from build123d import *

# Parameters (mm, degrees)
SKETCH3_R           = 3.9
BOSS_EXTRUDE1_DEPTH = 5
SKETCH5_R           = 3.6
BOSS_EXTRUDE2_DEPTH = 5
BOSS_EXTRUDE3_DEPTH = 5
SKETCH7_R           = 1.25
CUT_EXTRUDE1_DEPTH  = 11


with BuildPart() as part:
    # Sketch3 → Boss-Extrude1 (new body)
    with BuildSketch(Plane.XY):
        with Locations((10, 0)):
            Circle(SKETCH3_R)
        with BuildLine():
            Line((10, 2.1), (9.774921544, 2.489847322))
            ThreePointArc((9.774921544, 2.489847322), (9.608913837, 2.469220851), (9.444657197, 2.437538589))
            Line((9.444657197, 2.437538589), (9.351064312, 1.997218684))
            Line((9.351064312, 1.997218684), (9.016532531, 2.298432452))
            ThreePointArc((9.016532531, 2.298432452), (8.865023751, 2.22751631), (8.71859676, 2.146626594))
            Line((8.71859676, 2.146626594), (8.76565097, 1.698935688))
            Line((8.76565097, 1.698935688), (8.354412167, 1.882031))
            ThreePointArc((8.354412167, 1.882031), (8.232233047, 1.767766953), (8.117969, 1.645587833))
            Line((8.117969, 1.645587833), (8.301064312, 1.23434903))
            Line((8.301064312, 1.23434903), (7.853373406, 1.28140324))
            ThreePointArc((7.853373406, 1.28140324), (7.77248369, 1.134976249), (7.701567548, 0.983467469))
            Line((7.701567548, 0.983467469), (8.002781316, 0.648935688))
            Line((8.002781316, 0.648935688), (7.562461411, 0.555342803))
            ThreePointArc((7.562461411, 0.555342803), (7.530779149, 0.391086163), (7.510152678, 0.225078456))
            Line((7.510152678, 0.225078456), (7.9, 0))
            Line((7.9, 0), (7.510152678, -0.225078456))
            ThreePointArc((7.510152678, -0.225078456), (7.530779149, -0.391086163), (7.562461411, -0.555342803))
            Line((7.562461411, -0.555342803), (8.002781316, -0.648935688))
            Line((8.002781316, -0.648935688), (7.701567548, -0.983467469))
            ThreePointArc((7.701567548, -0.983467469), (7.77248369, -1.134976249), (7.853373406, -1.28140324))
            Line((7.853373406, -1.28140324), (8.301064312, -1.23434903))
            Line((8.301064312, -1.23434903), (8.117969, -1.645587833))
            ThreePointArc((8.117969, -1.645587833), (8.232233047, -1.767766953), (8.354412167, -1.882031))
            Line((8.354412167, -1.882031), (8.76565097, -1.698935688))
            Line((8.76565097, -1.698935688), (8.71859676, -2.146626594))
            ThreePointArc((8.71859676, -2.146626594), (8.865023751, -2.22751631), (9.016532531, -2.298432452))
            Line((9.016532531, -2.298432452), (9.351064312, -1.997218684))
            Line((9.351064312, -1.997218684), (9.444657197, -2.437538589))
            ThreePointArc((9.444657197, -2.437538589), (9.608913837, -2.469220851), (9.774921544, -2.489847322))
            Line((9.774921544, -2.489847322), (10, -2.1))
            Line((10, -2.1), (10.225078456, -2.489847322))
            ThreePointArc((10.225078456, -2.489847322), (10.391086163, -2.469220851), (10.555342803, -2.437538589))
            Line((10.555342803, -2.437538589), (10.648935688, -1.997218684))
            Line((10.648935688, -1.997218684), (10.983467469, -2.298432452))
            ThreePointArc((10.983467469, -2.298432452), (11.134976249, -2.22751631), (11.28140324, -2.146626594))
            Line((11.28140324, -2.146626594), (11.23434903, -1.698935688))
            Line((11.23434903, -1.698935688), (11.645587833, -1.882031))
            ThreePointArc((11.645587833, -1.882031), (11.767766953, -1.767766953), (11.882031, -1.645587833))
            Line((11.882031, -1.645587833), (11.698935688, -1.23434903))
            Line((11.698935688, -1.23434903), (12.146626594, -1.28140324))
            ThreePointArc((12.146626594, -1.28140324), (12.22751631, -1.134976249), (12.298432452, -0.983467469))
            Line((12.298432452, -0.983467469), (11.997218684, -0.648935688))
            Line((11.997218684, -0.648935688), (12.437538589, -0.555342803))
            ThreePointArc((12.437538589, -0.555342803), (12.469220851, -0.391086163), (12.489847322, -0.225078456))
            Line((12.489847322, -0.225078456), (12.1, 0))
            Line((12.1, 0), (12.489847322, 0.225078456))
            ThreePointArc((12.489847322, 0.225078456), (12.469220851, 0.391086163), (12.437538589, 0.555342803))
            Line((12.437538589, 0.555342803), (11.997218684, 0.648935688))
            Line((11.997218684, 0.648935688), (12.298432452, 0.983467469))
            ThreePointArc((12.298432452, 0.983467469), (12.22751631, 1.134976249), (12.146626594, 1.28140324))
            Line((12.146626594, 1.28140324), (11.698935688, 1.23434903))
            Line((11.698935688, 1.23434903), (11.882031, 1.645587833))
            ThreePointArc((11.882031, 1.645587833), (11.767766953, 1.767766953), (11.645587833, 1.882031))
            Line((11.645587833, 1.882031), (11.23434903, 1.698935688))
            Line((11.23434903, 1.698935688), (11.28140324, 2.146626594))
            ThreePointArc((11.28140324, 2.146626594), (11.134976249, 2.22751631), (10.983467469, 2.298432452))
            Line((10.983467469, 2.298432452), (10.648935688, 1.997218684))
            Line((10.648935688, 1.997218684), (10.555342803, 2.437538589))
            ThreePointArc((10.555342803, 2.437538589), (10.391086163, 2.469220851), (10.225078456, 2.489847322))
            Line((10.225078456, 2.489847322), (10, 2.1))
        make_face(mode=Mode.SUBTRACT)
    extrude(amount=-BOSS_EXTRUDE1_DEPTH)

    # Sketch5 → Boss-Extrude2 (add)
    with BuildSketch(Plane(origin=(0, 0, -5), x_dir=(-1, 0, 0), z_dir=(0, 0, -1))):
        with Locations((-10, 0)):
            Circle(SKETCH5_R)
    extrude(amount=BOSS_EXTRUDE2_DEPTH)

    # Sketch6 → Boss-Extrude3 (add)
    with BuildSketch(Plane(origin=(0, 0, -10), x_dir=(-1, 0, 0), z_dir=(0, 0, -1))):
        with BuildLine():
            ThreePointArc((-13.070257041, -1.879766396), (-12.89955723, 2.133674734), (-9.118539931, 3.49041948))
            Line((-9.118539931, 3.49041948), (-12.569087005, 5.118573235))
            Line((-12.569087005, 5.118573235), (-15.65106162, 0.930323902))
            Line((-15.65106162, 0.930323902), (-13.070257041, -1.879766396))
        make_face()
    extrude(amount=-BOSS_EXTRUDE3_DEPTH)

    # Sketch7 → Cut-Extrude1 (cut, through all)
    with BuildSketch(Plane(origin=(0, 0, -10), x_dir=(-1, 0, 0), z_dir=(0, 0, -1))):
        with Locations((-10, 0)):
            Circle(SKETCH7_R)
    extrude(amount=-CUT_EXTRUDE1_DEPTH, mode=Mode.SUBTRACT)


solid = part.part
Work out the finished part from the listing and answer in its coordinate system (mm). A direction names the side the tool comes from. Give positions to 0.01 mm unless a question says otherwise; leave off trailing zeros. Loops run counter-clockwise (first coordinate to the right, second up) from the corner with the lowest first, then second, coordinate; pieces in that order, holes last. Notation, with made-up numbers: (87, -9) -> (143, -9) arc R34 cw to (143, 27) -> close; hole circle Ø10 at (15, 44). An arc over 180 degrees is marked (long way). Use a Markdown table: item, result. Add a question column.
1. Section B-B on y = 3.75 is taken. Determine the outline of the cut face in (x, z), and give its area (3 significant figures).
2. Section C-C on x = 11.5 is taken. Determine the outline of the cut face in (y, z).
3. Section D-D on x = 13.5 is taken. Determine the outline of the cut face in (y, z), and give its area (3 significant figures).
4. Find the intervals of material crossed by probe 1 along Z at (x, y) = (9.25, 1.75); probe 2 along X at (y, z) = (-0.5, -8.5); probe 3 along Y at (x, z) = (10, -7.9), in increasing order.
5. Flat-ended cylindrical pins translate along their axes: pin 1 Ø1 at (x, z) = (12, -4) entering from -Y; pin 2 Ø3 at (x, y) = (10, 0) entering from +Z. Find the tip coordinate at first contact, or state that the pin passes through.
6. Section A-A on z = -9 is taken. Determine the outline of the cut face in (x, y), and give its area (3 significant figures).
7. Determine the mould class of faces 6 (the cylindrical face through (6.104, 0.171, -2.465)), 7 (the flat face through (13, 3, -5)), 8 (the flat face through (9, 1, -5)), 9 (the cylindrical face through (11.25, 0.05, -7.54)) for opening direction Y: released by +Y, released by -Y, zero draft, split by the parting line, or undercut.
8. For faces 1 (the flat face through (10.82, 4.293, -7.535)), 2 (the flat face through (14.379, -0.455, -7.535)), 3 (the flat face through (14.09, 3.05, -7.54)), 4 (the cylindrical face through (7.16, -2.21, -7.46)), 5 (the flat face through (10, -3, 0)), determine the directions among +Z, -Z, +X, -X, +Y, -Y from which every point of the face is accessible in a straight line to the end or side of a thin tool.
Results below:
| question | item | result |
|---|---|---|
| 1 | outline | (8.93, -5) -> (9.67, -5) -> (9.67, -10) -> (13.58, -10) -> (13.58, -5) -> (11.07, -5) -> (11.07, 0) -> (8.93, 0) -> close |
| 1 | area | 30.2 mm^2 |
| 2 | outline | (-3.6, -5) -> (-3.27, -5) -> (-3.27, -10) -> (4.61, -10) -> (4.61, -5) -> (3.6, -5) -> (3.6, 0) -> (1.82, 0) -> (1.82, -5) -> (-1.82, -5) -> (-1.82, 0) -> (-3.6, 0) -> close |
| 3 | outline | (-1.72, -5) -> (-1.41, -5) -> (-1.41, -10) -> (3.85, -10) -> (3.85, -5) -> (1.72, -5) -> (1.72, 0) -> (-1.72, 0) -> close |
| 3 | area | 43.5 mm^2 |
| 4 | probe 1 | z = -10 to -5 |
| 4 | probe 2 | x = 6.43 to 8.85, 11.15 to 14.34 |
| 4 | probe 3 | y = -3.6 to -1.25, 1.25 to 3.91 |
| 5 | pin 1 | stops at y = -3.6 |
| 5 | pin 2 | stops at z = -5 |
| 6 | outline | (9.12, 3.49) arc R3.6 ccw (long way) to (13.07, -1.88) -> (15.65, 0.93) -> (12.57, 5.12) -> close; hole circle Ø2.5 at (10, 0) |
| 6 | area | 47.2 mm^2 |
| 7 | face 6 | split by the parting line |
| 7 | face 7 | zero draft |
| 7 | face 8 | undercut |
| 7 | face 9 | undercut |
| 8 | face 1 | -Z, -X, +Y |
| 8 | face 2 | -Z, +X, -Y |
| 8 | face 3 | +Z, -Z, +X, +Y |
| 8 | face 4 | -Z |
| 8 | face 5 | +Z, +X, -X, +Y, -Y |
